```python
from build123d import *

# Parameters (mm, degrees)
IZIM1_R                     = 40
Y_KSEKLIK_EKSTR_ZYON1_DEPTH = 120
IZIM2_R                     = 10
KES_EKSTR_ZYON1_DEPTH       = 30
KUBBE1_FACE_RADIUS          = 40
KUBBE1_HEIGHT               = 20


with BuildPart() as part:
    # Çizim1 → Yükseklik-Ekstrüzyon1 (new body)
    with BuildSketch(Plane.XY):
        Circle(IZIM1_R)
    extrude(amount=Y_KSEKLIK_EKSTR_ZYON1_DEPTH)

    # Çizim2 → Kes-Ekstrüzyon1 (cut)
    with BuildSketch(Plane(origin=(0, 20, 0), x_dir=(1, 0, 0), z_dir=(0, 1, 0))):
        with Locations(Location((0, -100, 0), (0, 0, 90))):
            Circle(IZIM2_R)
    kes_ekstr_zyon1 = extrude(amount=KES_EKSTR_ZYON1_DEPTH, mode=Mode.SUBTRACT)

    # Aynalama1: Kes-Ekstrüzyon1 across plane
    add(kes_ekstr_zyon1.mirror(Plane.ZX), mode=Mode.SUBTRACT)

    # Kubbe1: a dome of height H over a round flat face of radius A is a cap of a sphere of radius (A * A + H * H) / (2 * H)
    kubbe1_r = (KUBBE1_FACE_RADIUS * KUBBE1_FACE_RADIUS + KUBBE1_HEIGHT * KUBBE1_HEIGHT) / (2 * KUBBE1_HEIGHT)
    kubbe1_base = Plane((0, 0, 120), z_dir=(0, 0, 1))
    with Locations(kubbe1_base.offset(KUBBE1_HEIGHT - kubbe1_r)):
        kubbe1_ball = Sphere(kubbe1_r, mode=Mode.PRIVATE)
    add(split(kubbe1_ball, bisect_by=kubbe1_base, keep=Keep.TOP, mode=Mode.PRIVATE))


solid = part.part
```
The listing builds one solid part. Answer for the finished solid, in the listing's coordinates (mm). A direction names the side the tool comes from. Round coordinates to 2 decimals unless told otherwise and drop trailing zeros. Write each loop counter-clockwise with the first axis right and the second up, starting at its lowest first coordinate (ties: lowest second). Pieces come first, ordered by that corner, then holes. Notation, with made-up numbers: (44.5, -11) -> (59.5, -11) arc R15 ccw to (59.5, 9) -> close; hole circle Ø2 at (-9.75, 38.5). An arc over 180 degrees is marked (long way). Write item = value, one per line.
1) Section A-A on z = 100 is taken. Write down the section's boundary in (x, y).
Check values:
outline = (-10, -38.73) -> (-10, -20) -> (10, -20) -> (10, -38.73) arc R40 ccw to (10, 38.73) -> (10, 20) -> (-10, 20) -> (-10, 38.73) arc R40 ccw to start
2) Straight lines are drawn through the part: line 1 along X through (y, z) = (-23.75, 100); line 2 along X through (y, z) = (33, 100); line 3 along Z through (x, y) = (-8, 31). For each, find the intervals that lie inside material, in ascending order. Write a range as [from, to].
Check values:
line_1 = [-32.19, -10], [10, 32.19]
line_2 = [-22.61, -10], [10, 22.61]
line_3 = [0, 94], [106, 128.41]
3) Which of the six approach directions +Z, -Z, +X, -X, +Y, -Y give full straight-line access (tool end or side, diameter ignored) to faces 1 (the cylindrical face through (38.153, 12.015, 59.16)), 2 (the cylindrical face through (9.76, -29.87, 102.17)), 3 (the flat face through (0, 20, 100))?
Check values:
face_1 = +Z, -Z
face_2 = -Y
face_3 = +Y
4) Section D-D on y = 0 is taken. Write down the section's boundary in (x, z).
Check values:
outline = (-40, 0) -> (40, 0) -> (40, 120) arc R50 ccw to (-40, 120) -> close
5) Section C-C on x = -1.5 is taken. Write down the section's boundary in (y, z), plus the area to 3 significant figures.
Check values:
outline = (-39.97, 0) -> (39.97, 0) -> (39.97, 90.11) -> (20, 90.11) -> (20, 109.89) -> (39.97, 109.89) -> (39.97, 120) arc R49.98 ccw to (-39.97, 120) -> (-39.97, 109.89) -> (-20, 109.89) -> (-20, 90.11) -> (-39.97, 90.11) -> close
area = 9,920 mm²
6) Section B-B on y = 21.5 is taken. Write down the section's boundary in (x, z), plus the area to 3 significant figures.
Check values:
outline = (-33.73, 0) -> (33.73, 0) -> (33.73, 120) arc R45.14 ccw to (-33.73, 120) -> close; hole circle Ø20 at (0, 100)
area = 8,490 mm²
7) For a pull along Z with two mould halves and no side action, classify faces 4 (the flat face through (0, -20, 100)), 5 (the flat face through (-1, 1, 0)) as released by +Z, released by -Z, zero draft, split by the parting line, or undercut.
Check values:
face_4 = undercut
face_5 = released by -Z
8) Given pin 1 (6 mm diameter, centred on x = 25.5, y = 5, fed in from -Z); pin 2 (6 mm diameter, centred on x = -3, z = 96, fed in from +Y); pin 3 (6 mm diameter, centred on y = -30, z = 66.5, fed in from -X); pin 4 (10 mm diameter, centred on x = -25, y = -23.5, fed in from +Z), each flat-ended and moving along its own axis, determine where each tip first touches the part or whether it passes through.
Check values:
pin_1 = 0
pin_2 = 20
pin_3 = -29.51
pin_4 = 130.51
